```python
from build123d import *

# Parameters (mm, degrees)
SKETCH_1_W          = 127.26
SKETCH_1_H          = 80
EXTRUDE_1_DEPTH     = 2
EXTRUDE_2_DEPTH     = 2
SKETCH_3_R          = 1.625
SKETCH_3_R_2        = 1.65
CUT_EXTRUDE_1_DEPTH = 32


with BuildPart() as part:
    # 草图1 → 凸台-拉伸1 (new body)
    with BuildSketch(Plane.XY):
        Rectangle(SKETCH_1_W, SKETCH_1_H)
    extrude(amount=EXTRUDE_1_DEPTH)

    # 草图2 → 凸台-拉伸2 (add)
    with BuildSketch(Plane(origin=(0, 0, 0), x_dir=(-1, 0, 0), z_dir=(0, 0, -1))):
        Polygon((143.63, 40), (63.63, 40), (63.63, -40), (91.914271247, -40), (157.772135624, 25.857864376), align=None)
        Polygon((-63.63, -40), (-63.63, 40), (-143.63, 40), (-157.772135624, 25.857864376), (-91.914271247, -40), align=None)
    extrude(amount=-EXTRUDE_2_DEPTH)

    # 草图3 → 切除-拉伸1 (cut)
    with BuildSketch(Plane.XY.offset(2)):
        with Locations((-50, 12)):
            Circle(SKETCH_3_R)
        with Locations((-50, -18)):
            Circle(SKETCH_3_R)
        with Locations((50, 12)):
            Circle(SKETCH_3_R)
        with Locations((50, -18)):
            Circle(SKETCH_3_R)
        with Locations((-122.416796564, 4.644660941)):
            Circle(SKETCH_3_R)
        with Locations((-96.960952442, -20.811183182)):
            Circle(SKETCH_3_R)
        with Locations((96.960952442, -20.811183182)):
            Circle(SKETCH_3_R)
        with Locations((122.416796564, 4.644660941)):
            Circle(SKETCH_3_R)
        with Locations((-75, 30)):
            Circle(SKETCH_3_R_2)
        with Locations((75, 30)):
            Circle(SKETCH_3_R_2)
        Polygon((80.600562748, -25.857864376), (74.943708499, -20.201010127), (55.144718626, -40), (66.458427125, -40), align=None)
        Polygon((-106.914271247, -25), (-92.772135624, -25), (-77.772135624, -40), (-106.914271247, -40), align=None)
        Polygon((-133.023398282, 1.109127035), (-113.63, 20.502525317), (-113.63, 40), (-143.63, 40), (-157.772135624, 25.857864376), align=None)
        Polygon((157.772135624, 25.857864376), (133.023398282, 1.109127035), (113.63, 20.502525317), (113.63, 40), (143.63, 40), align=None)
    extrude(amount=-CUT_EXTRUDE_1_DEPTH, mode=Mode.SUBTRACT)


solid = part.part
```
Here's how the part is built. I have some questions about the finished solid (model axes, mm). A direction names the side the tool comes from. Give positions to 0.01 mm unless a question says otherwise; leave off trailing zeros. Write each loop counter-clockwise with the first axis right and the second up, starting at its lowest first coordinate (ties: lowest second). Pieces come first, ordered by that corner, then holes. Notation, with made-up numbers: M -35,61 L 18,61 A18 ccw 18,76 Z; hole C -6.5,-31.5 d5. An arc over 180 degrees is marked long. Put each result on its own line as item: value. Start each with the question number.
Item 1: Will these pins go through, and if not, where does the flat tip stop? pin 1 (0.6 mm diameter, centred on y = 27.5, z = 1, fed in from -X); pin 2 (1 mm diameter, centred on y = 32, z = 2, fed in from +X); pin 3 (1 mm diameter, centred on x = -98, z = 1, fed in from -Y).
Item 2: On a 3-axis mill with a long thin cutter (end or side, diameter ignored), from which of +Z, -Z, +X, -X, +Y, -Y can I reach the whole of each face in a straight line? I mean faces 1 (the flat face through (73.43, -33.03, 1.01)), 2 (the flat face through (112.757, -19.158, 0.986)). Say none if no direction works.
Item 3: If we section it at B-B, the plane y = -13: Write out the boundary of the cut face in (x, z), then the cut area to 3 significant figures.
Item 4: If we section it at A-A, the plane z = 1.2: Count the separate pieces of the cut face and the enclosed holes in it, then the cut area to 3 significant figures.
Item 5: I need wall thicknesses on L1, parallel to Y at x = 50, z = 0.95 (3 decimals); L2, parallel to Y at x = -75, z = 0.4; L3, parallel to Y at x = 75, z = 1.4. Which ranges of each line are inside material? Lowest first, please. Write a range as from..to.
Item 6: Thinking about a two-plate mould opening in Y: for faces 3 (the flat face through (-123.46, 10.67, 1.01)), 4 (the flat face through (2, 1, 0)), 5 (the flat face through (65.183, -29.962, 1.014)), which applies, +Y half, -Y half, draft (parallel to the pull), parting line (faces both ways), or undercut?
Values:
1. pin 1: x = -113.63
1. pin 2: x = 113.63
1. pin 3: y = -25
2. face 1: +Z, -Z
2. face 2: +Z, -Z, +X, -Y
3. outline: M -118.91,0 L 118.91,0 L 118.91,2 L -118.91,2 Z
3. area: 476 mm²
4. separate pieces: 1
4. enclosed holes: 10
4. area: 18,000 mm²
5. L1: -40..-19.625, -16.375..10.375, 13.625..40
5. L2: -40..28.35, 31.65..40
5. L3: -40..-31.46, -20.26..28.35, 31.65..40
6. face 3: +Y half
6. face 4: draft
6. face 5: undercut
